CAD build for the part. Positions are in the model's coordinates, mm. Face numbers are marked on the shaded views. A direction names the side the tool comes from. Give positions to 0.01 mm unless a question says otherwise; leave off trailing zeros. Write each loop counter-clockwise with the first axis right and the second up, starting at its lowest first coordinate (ties: lowest second). Pieces come first, ordered by that corner, then holes. Notation, with made-up numbers: (-9.5, 38) - (6.5, 38) arc R14 cw to (6.5, 65) - close; hole circle Ø8 at (72.25, 4.5). An arc over 180 degrees is marked (long way). Put each result on its own line as item: value. Start each with the question number.
1. Cut at B-B on z = -1. List the corners of the cut face in (x, y), and give its area (3 significant figures).
2. Cut at D-D on z = 11.25. List the corners of the cut face in (x, y).
3. Wall check: line 1 (Z direction, x = 0, y = 4.25); line 2 (X direction, y = 4, z = 14); line 3 (Z direction, x = 0.25, y = 2.25). Give the ranges that are in metal, low to high.
4. Drop flat-ended pins along their axis: pin 1 (2 mm diameter, centred on x = 0, z = -0.46, fed in from -Y); pin 2 (1.9 mm diameter, centred on y = 4, z = 14, fed in from +X); pin 3 (1.9 mm diameter, centred on y = 4, z = 14.5, fed in from -X). Give the stop position or say it passes through.
5. Cut at A-A on x = 0. List the corners of the cut face in (y, z).
6. Tool access for the marked faces 4, 5 and 6: list every direction of +Z, -Z, +X, -X, +Y, -Y with a clear straight run to the whole face (end or side of a thin tool).
7. Cut at C-C on y = 2.75. List the corners of the cut face in (x, z), and give its area (3 significant figures).
8. Mould opens along X. For the marked faces 1, 2 and 3 say: +X half, -X half, draft (parallel to the pull), parting line (faces both ways), or undercut.
from build123d import *

# Parameters (mm, degrees)
BOSS_EXTRUDE1_DEPTH   = 6.35
F_6_CLEARANCE_HOLE1_D = 3.6576


with BuildPart() as part:
    # Sketch1 → Boss-Extrude1 (new body)
    with BuildSketch(Plane(origin=(0, 0, 0), x_dir=(1, 0, 0), z_dir=(0, 1, 0))):
        Polygon((-15, -10), (-15, 10), (15, 10), (15, -10), (11.82, -10), (11.82, -16.35), (-11.82, -16.35), (-11.82, -10), align=None)
    extrude(amount=BOSS_EXTRUDE1_DEPTH)

    # #6 Clearance Hole1 (through all)
    with Locations(Plane(origin=(0, 6.35, 0), x_dir=(1, 0, 0), z_dir=(0, 1, 0))):
        with Locations((0, 0.4648)):
            Hole(F_6_CLEARANCE_HOLE1_D / 2)


solid = part.part
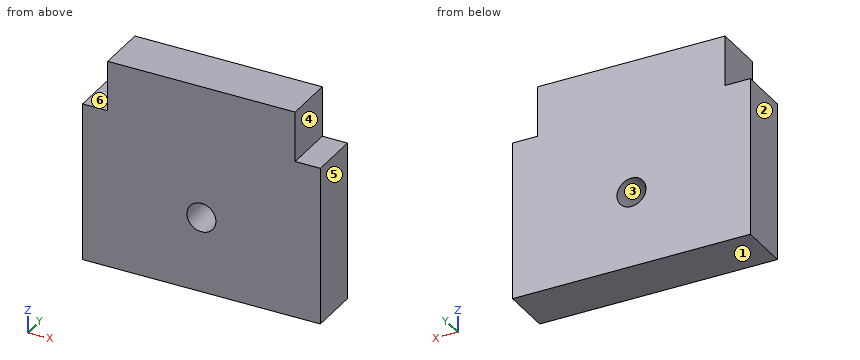
Report:
1. outline: (-15, 0) - (-1.75, 0) - (-1.75, 6.35) - (-15, 6.35) - close; (1.75, 0) - (15, 0) - (15, 6.35) - (1.75, 6.35) - close
1. area: 168 mm²
2. outline: (-11.82, 0) - (11.82, 0) - (11.82, 6.35) - (-11.82, 6.35) - close
3. line 1: z = -10 to -2.29, 1.36 to 16.35
3. line 2: x = -11.82 to 11.82
3. line 3: z = -10 to -2.28, 1.35 to 16.35
4. pin 1: passes through
4. pin 2: stops at x = 11.82
4. pin 3: stops at x = -11.82
5. outline: (0, -10) - (6.35, -10) - (6.35, -2.29) - (0, -2.29) - close; (0, 1.36) - (6.35, 1.36) - (6.35, 16.35) - (0, 16.35) - close
6. face 4: +Z, +X, +Y, -Y
6. face 5: +Z, -Z, +X, +Y, -Y
6. face 6: +Z, -X, +Y, -Y
7. outline: (-15, -10) - (15, -10) - (15, 10) - (11.82, 10) - (11.82, 16.35) - (-11.82, 16.35) - (-11.82, 10) - (-15, 10) - close; hole circle Ø3.66 at (0, -0.46)
7. area: 740 mm²
8. face 1: draft
8. face 2: -X half
8. face 3: undercut
